Part model, mm, in its own coordinate system. A direction names the side the tool comes from. Round coordinates to 2 decimals unless told otherwise and drop trailing zeros. Order: outer loops, then holes, each group sorted by start corner. A loop starts at its lowest first (then second) coordinate and runs counter-clockwise, first axis right, second up. Notation, with made-up numbers: (68, -30) -> (118, -30) arc R19 cw to (118, -5) -> close; hole circle Ø4 at (48.5, 9.25). An arc over 180 degrees is marked (long way). Answer as a JSON object with one key per item and string values. Group by question number.
```python
from build123d import *

# Parameters (mm, degrees)
SKETCH1_R               = 5
BOSS_EXTRUDE1_DEPTH     = 30
SKETCH1_3_R             = 5
CUT_EXTRUDE1_DEPTH      = 25
CHAMFER1_SIZE           = 0.75
SKETCH3_W               = 10
SKETCH3_H               = 5
SKETCH7_R               = 6.1
BOSS_EXTRUDE3_DEPTH     = 2.5
BOSS_EXTRUDE3_TAPER     = 45
CUT_EXTRUDE3_DEPTH      = 51.39841282
CUT_EXTRUDE3_DEPTH_BACK = 200
SKETCH8_R               = 2.5


with BuildPart() as part:
    # Sketch1 → Boss-Extrude1 (new body)
    # profile 1 of 2: a face of its own
    with BuildSketch(Plane(origin=(0, 0, 0), x_dir=(0, 0, -1), z_dir=(1, 0, 0))):
        with BuildLine():
            Line((2.5, 6.5), (-2.5, 6.5))
            ThreePointArc((-2.5, 6.5), (-5.328427125, 5.328427125), (-6.5, 2.5))
            Line((-6.5, 2.5), (-6.5, -2.5))
            ThreePointArc((-6.5, -2.5), (-5.328427125, -5.328427125), (-2.5, -6.5))
            Line((-2.5, -6.5), (2.5, -6.5))
            ThreePointArc((2.5, -6.5), (5.328427125, -5.328427125), (6.5, -2.5))
            Line((6.5, -2.5), (6.5, 2.5))
            ThreePointArc((6.5, 2.5), (5.328427125, 5.328427125), (2.5, 6.5))
        make_face()
        Circle(SKETCH1_R, mode=Mode.SUBTRACT)
    # profile 2 of 2: a face of its own
    with BuildSketch(Plane(origin=(0, 0, 0), x_dir=(0, 0, -1), z_dir=(1, 0, 0))):
        Circle(SKETCH1_R)
    extrude(amount=BOSS_EXTRUDE1_DEPTH)

    # Sketch1_3 → Cut-Extrude1 (cut)
    with BuildSketch(Plane(origin=(0, 0, 0), x_dir=(0, 0, -1), z_dir=(1, 0, 0))):
        Circle(SKETCH1_3_R)
    extrude(amount=CUT_EXTRUDE1_DEPTH, mode=Mode.SUBTRACT)

    # Chamfer1
    chamfer1_edges = [part.edges().sort_by_distance(p)[0] for p in [
        (0, 0, 5),
    ]]
    chamfer(chamfer1_edges, length=CHAMFER1_SIZE)

    # Sketch3 → Revolve2 (revolve)
    with BuildSketch(Plane(origin=(36, 0, 0), x_dir=(0, 0, -1), z_dir=(1, 0, 0))):
        with Locations((-5, 0)):
            Rectangle(SKETCH3_W, SKETCH3_H)
    revolve(axis=Axis((36, -11.950836094, 0), (0, 1, 0)))

    # Sketch4 → Revolve3 (revolve)
    with BuildSketch(Plane(origin=(36, 0, 0), x_dir=(0, 0, -1), z_dir=(1, 0, 0))):
        with BuildLine():
            Line((0, 2.5), (-10, 2.5))
            Line((-10, 2.5), (-10, 2.6))
            ThreePointArc((-10, 2.6), (-8.857716447, 5.357716447), (-6.1, 6.5))
            Line((-6.1, 6.5), (0, 6.5))
            Line((0, 6.5), (0, 2.5))
        make_face()
    revolve3 = revolve(axis=Axis((36, -7.102905922, 0), (0, 1, 0)))

    # Mirror3: Revolve3 across plane
    add(revolve3.mirror(Plane.ZX))

    # Sketch7 → Boss-Extrude3 (add)
    with BuildSketch(Plane(origin=(0, 6.5, 0), x_dir=(1, 0, 0), z_dir=(0, 1, 0))):
        with Locations((36, 0)):
            Circle(SKETCH7_R)
    boss_extrude3 = extrude(amount=BOSS_EXTRUDE3_DEPTH, taper=BOSS_EXTRUDE3_TAPER)

    # Mirror5: Boss-Extrude3 across plane
    add(boss_extrude3.mirror(Plane.ZX))

    # Sketch8 → Cut-Extrude3 (cut, two sides: drawn at the far end of the back side and taken through both)
    with BuildSketch(Plane(origin=(0, 9, 0), x_dir=(1, 0, 0), z_dir=(0, 1, 0)).offset(-CUT_EXTRUDE3_DEPTH_BACK)):
        with Locations(Location((36, 0, 0), (0, 0, 90))):
            Circle(SKETCH8_R)
    extrude(amount=CUT_EXTRUDE3_DEPTH + CUT_EXTRUDE3_DEPTH_BACK, mode=Mode.SUBTRACT)


solid = part.part
```
Q1. Drop flat-ended pins along their axis: pin 1 Ø2.5 at (x, z) = (13.5, 0) entering from -Y; pin 2 Ø6 at (x, z) = (25, -7.5) entering from +Y; pin 3 Ø1 at (x, y) = (34.5, 3.5) entering from +Z. Give the stop position or say it passes through.
Q2. Which spindle directions (+Z, -Z, +X, -X, +Y, -Y) get a long thin tool onto all of the face, cutting with end or side? Do faces 4 (the cylindrical face through (14.79, 5.297, -5.359)), 5 (the cylindrical face through (14.79, -5.359, -5.297)), 6 (the flat face through (14, 0, 6.5)), 7 (the flat face through (14, 0, -6.5)), 8 (the flat face through (25, 0, 0)). Say none if no direction does.
Q3. Band-saw the part on A-A (x = 36). List the corners of the cut face in (y, z), plus the area to 3 significant figures.
Q4. Band-saw the part on B-B (y = 0). List the corners of the cut face in (x, z).
Q5. Wall check: line 1 (Y direction, x = 8.25, z = 0); line 2 (X direction, y = -3.75, z = 0); line 3 (Z direction, x = 27, y = 0). Give the ranges that are in metal, low to high. Write a range as [from, to].
Q6. Band-saw the part on C-C (x = 16). List the corners of the cut face in (y, z).
Q7. Band-saw the part on D-D (y = -7.25). List the corners of the cut face in (x, z).
Q8. Two-plate mould, pull along Y, no slides. Class faces 1 (the cylindrical face through (12.71, -4.88, 1.08)), 2 (the cylindrical face through (14.79, -5.297, 5.359)), 3 (the cylindrical face through (33.89, -0.13, -1.34)): +Y half, -Y half, draft (parallel to the pull), parting line (faces both ways), or undercut.
Completed:
{
 "1": {"pin 1": "y = -6.5", "pin 2": "y = 5.96", "pin 3": "z = 9.9"},
 "2": {"face 4": "-Z, -X, +Y", "face 5": "-Z, -X, -Y", "face 6": "+Z, -X, +Y, -Y", "face 7": "-Z, -X, +Y, -Y", "face 8": "-X"},
 "3": {"outline": "(-9, -3.6) -> (-6.5, -6.1) arc R3.9 ccw to (-2.6, -10) -> (2.6, -10) arc R3.9 ccw to (6.5, -6.1) -> (9, -3.6) -> (9, -2.5) -> (-9, -2.5) -> close; (-9, 2.5) -> (9, 2.5) -> (9, 3.6) -> (6.5, 6.1) arc R3.9 ccw to (2.6, 10) -> (-2.6, 10) arc R3.9 ccw to (-6.5, 6.1) -> (-9, 3.6) -> close", "area": "205 mm2"},
 "4": {"outline": "(0, -6.5) -> (28.4, -6.5) arc R10 ccw (long way) to (28.4, 6.5) -> (0, 6.5) -> (0, 5.75) -> (0.75, 5) -> (25, 5) -> (25, -5) -> (0.75, -5) -> (0, -5.75) -> close; hole circle Ø5 at (36, 0)"},
 "5": {"line 1": "[-6.5, -5], [5, 6.5]", "line 2": "[25, 33.5], [38.5, 45.83]", "line 3": "[-6.5, 6.5]"},
 "6": {"outline": "(-6.5, -2.5) arc R4 ccw to (-2.5, -6.5) -> (2.5, -6.5) arc R4 ccw to (6.5, -2.5) -> (6.5, 2.5) arc R4 ccw to (2.5, 6.5) -> (-2.5, 6.5) arc R4 ccw to (-6.5, 2.5) -> close; hole circle Ø10 at (0, 0)"},
 "7": {"outline": "circle Ø10.7 at (36, 0); hole circle Ø5 at (36, 0)"},
 "8": {"face 1": "undercut", "face 2": "-Y half", "face 3": "draft"}
}
